Part model, mm, in its own coordinate system. A direction names the side the tool comes from. Give positions to 0.01 mm unless a question says otherwise; leave off trailing zeros. Write each loop counter-clockwise with the first axis right and the second up, starting at its lowest first coordinate (ties: lowest second). Pieces come first, ordered by that corner, then holes.
from build123d import *

# Parameters (mm, degrees)
P_IDAT_VYSUNUT_M1_DEPTH  = 14.05
P_IDAT_VYSUNUT_M2_DEPTH  = 1.5
ODEBRAT_VYSUNUT_M1_DEPTH = 1.6
ODEBRAT_VYSUNUT_M2_REACH = 454.909
SKICA4_R                 = 1.5


with BuildPart() as part:
    # Skica1 → Přidat vysunutím1 (new body)
    with BuildSketch(Plane.XY):
        Polygon((-1.7, 1.7), (429.98, 1.7), (429.98, -127.624163056), (423.673791129, -133.930371927), (415.733791129, -133.930371927), (413.350841277, -136.313321779), (14.929158723, -136.313321779), (12.546208871, -133.930371927), (4.606208871, -133.930371927), (-1.7, -127.624163056), align=None)
        Polygon((-0.1, 0.1), (428.38, 0.1), (428.38, -126.961421356), (423.01104943, -132.330371927), (415.07104943, -132.330371927), (412.688099577, -134.713321779), (15.591900423, -134.713321779), (13.20895057, -132.330371927), (5.26895057, -132.330371927), (-0.1, -126.961421356), align=None, mode=Mode.SUBTRACT)
    extrude(amount=-P_IDAT_VYSUNUT_M1_DEPTH)

    # Skica2 → Přidat vysunutím2 (add)
    with BuildSketch(Plane.XY):
        Polygon((-1.7, 1.7), (-1.7, -127.624163056), (4.606208871, -133.930371927), (12.546208871, -133.930371927), (14.929158723, -136.313321779), (413.350841277, -136.313321779), (415.733791129, -133.930371927), (423.673791129, -133.930371927), (429.98, -127.624163056), (429.98, 1.7), align=None)
        Polygon((4.3, -4.3), (4.3, -125.138881682), (7.091490245, -127.930371927), (15.031490245, -127.930371927), (17.414440098, -130.313321779), (410.865559902, -130.313321779), (413.248509755, -127.930371927), (421.188509755, -127.930371927), (423.98, -125.138881682), (423.98, -4.3), align=None, mode=Mode.SUBTRACT)
    extrude(amount=P_IDAT_VYSUNUT_M2_DEPTH)

    # Skica3 → Odebrat vysunutím1 (cut)
    with BuildSketch(Plane(origin=(0, 1.7, 0), x_dir=(1, 0, 0), z_dir=(0, 1, 0))):
        with BuildLine():
            Line((45.76, 5.7), (40.26, 5.7))
            ThreePointArc((40.26, 5.7), (36.71, 9.25), (40.26, 12.8))
            Line((40.26, 12.8), (45.76, 12.8))
            ThreePointArc((45.76, 12.8), (49.31, 9.25), (45.76, 5.7))
        make_face()
    extrude(amount=-ODEBRAT_VYSUNUT_M1_DEPTH, mode=Mode.SUBTRACT)

    # Odebrat vysunutím2: up to this face of the body (flat: up to its plane)
    odebrat_vysunut_m2_end = Plane(part.part.faces().sort_by_distance((429.98, -62.962081528, -6.275))[0])
    # Skica4 → Odebrat vysunutím2 (cut, up to the picked face)
    with BuildSketch(Plane.ZY.offset(1.7), mode=Mode.PRIVATE) as odebrat_vysunut_m2_sk1:
        with Locations(Location((-9.05, -22.962081528, 0), (0, 0, 180))):
            Circle(SKICA4_R)
    odebrat_vysunut_m2_tool1 = split(extrude(odebrat_vysunut_m2_sk1.sketch, amount=-ODEBRAT_VYSUNUT_M2_REACH, mode=Mode.PRIVATE), bisect_by=odebrat_vysunut_m2_end, keep=Keep.BOTH, mode=Mode.PRIVATE)
    # Skica4 → Odebrat vysunutím2 (cut, up to the picked face)
    with BuildSketch(Plane.ZY.offset(1.7), mode=Mode.PRIVATE) as odebrat_vysunut_m2_sk2:
        with Locations(Location((-9.05, -102.962081528, 0), (0, 0, 180))):
            Circle(SKICA4_R)
    odebrat_vysunut_m2_tool2 = split(extrude(odebrat_vysunut_m2_sk2.sketch, amount=-ODEBRAT_VYSUNUT_M2_REACH, mode=Mode.PRIVATE), bisect_by=odebrat_vysunut_m2_end, keep=Keep.BOTH, mode=Mode.PRIVATE)
    add(odebrat_vysunut_m2_tool1.solids().sort_by(Axis((-1.7, -22.962082, -9.05), (1, 0, 0)))[0], mode=Mode.SUBTRACT)
    add(odebrat_vysunut_m2_tool2.solids().sort_by(Axis((-1.7, -102.962082, -9.05), (1, 0, 0)))[0], mode=Mode.SUBTRACT)


solid = part.part
1) Drill centre lines: L1, parallel to Y at x = 429.6, z = -9.05; L2, parallel to X at y = -4, z = -10.75; L3, parallel to Y at x = 387, z = -11. Where is each one in solid material? Low to high.
Check result:
L1: y = -128 to -104.46, -101.46 to -24.46, -21.46 to 1.7
L2: x = -1.7 to -0.1, 428.38 to 429.98
L3: y = -136.31 to -134.71, 0.1 to 1.7
2) Saw through at A-A (y = -86). Write the cut outline in (x, z).
Check result:
outline: (-1.7, -14.05) - (-0.1, -14.05) - (-0.1, 0) - (4.3, 0) - (4.3, 1.5) - (-1.7, 1.5) - close; (423.98, 0) - (428.38, 0) - (428.38, -14.05) - (429.98, -14.05) - (429.98, 1.5) - (423.98, 1.5) - close
3) 3-axis set-ups, long thin cutter, end or side, ignore diameter. For faces 4 (the flat face through (9, -133.93, -6)), 5 (the flat face through (213, -133, 1.5)), 6 (the flat face through (428.38, -63, -7)): which of +Z, -Z, +X, -X, +Y, -Y reach the whole face in a straight line?
Check result:
face 4: +Z, -Z, -X, -Y
face 5: +Z, +X, -X, +Y, -Y
face 6: -Z
4) Mould opens along X. For faces 1 (the flat face through (429.98, -64, -6)), 2 (the flat face through (213, -2, 0)), 3 (the flat face through (420, -133.93, -6)) say: +X half, -X half, draft (parallel to the pull), parting line (faces both ways), or undercut.
Check result:
face 1: +X half
face 2: undercut
face 3: draft
5) Flat gauge pin, fed straight in: P1, Ø6.5, axis at x = 10, z = -5, coming from the -Y side. Where does the tip first touch, or does it go through?
Check result:
P1: stops at y = -134.63
6) Saw through at B-B (x = 242). Write the cut outline in (y, z), and give its area (3 significant figures).
Check result:
outline: (-136.31, -14.05) - (-134.71, -14.05) - (-134.71, 0) - (-130.31, 0) - (-130.31, 1.5) - (-136.31, 1.5) - close; (-4.3, 0) - (0.1, 0) - (0.1, -14.05) - (1.7, -14.05) - (1.7, 1.5) - (-4.3, 1.5) - close
area: 63.0 mm2
